```python
from build123d import *

# Parameters (mm, degrees)
BOSS_EXTRUDE1_DEPTH       = 12.7
FILLET1_R                 = 6.35
F_1_4_CLEARANCE_HOLE1_D   = 6.7564
TAP_DRILL_FOR_8_32_TAP1_D = 3.4544


with BuildPart() as part:
    # Sketch1 → Boss-Extrude1 (new body)
    with BuildSketch(Plane.XY):
        Polygon((12.7, 15.875), (31.75, 15.875), (31.75, 28.575), (-31.75, 28.575), (-31.75, 15.875), (-12.7, 15.875), (-12.7, -15.875), (12.7, -15.875), align=None)
    extrude(amount=BOSS_EXTRUDE1_DEPTH)

    # Fillet1
    fillet1_edges = [part.edges().sort_by_distance(p)[0] for p in [
        (-12.7, 15.875, 6.35),
        (12.7, 15.875, 6.35),
    ]]
    fillet(fillet1_edges, radius=FILLET1_R)

    # 1/4 Clearance Hole1 (through all)
    with Locations(Plane.XY.offset(12.7)):
        with Locations((0, -6.35), (0, 12.7)):
            Hole(F_1_4_CLEARANCE_HOLE1_D / 2)

    # Tap Drill for #8-32 Tap1 (through all)
    with Locations(Plane(origin=(0, 15.875, 0), x_dir=(-1, 0, 0), z_dir=(0, -1, 0))):
        with Locations((-25.4, -6.35), (25.4, -6.35)):
            Hole(TAP_DRILL_FOR_8_32_TAP1_D / 2)


solid = part.part
```
Read the model definition and answer for the solid it produces. Units are mm, in the model's axes. A direction names the side the tool comes from. Coordinates: 2 decimals unless noted, no trailing zeros. Loops run counter-clockwise (first coordinate to the right, second up) from the corner with the lowest first, then second, coordinate; pieces in that order, holes last.
(1) The part is cut by section B-B (z = 10.5). Determine the outline of the cut face in (x, y) (3 decimals), and give its area (3 significant figures).
Solution:
outline: (-31.75, 15.875) - (-19.05, 15.875) arc R6.35 cw to (-12.7, 9.525) - (-12.7, -15.875) - (12.7, -15.875) - (12.7, 9.525) arc R6.35 cw to (19.05, 15.875) - (31.75, 15.875) - (31.75, 28.575) - (-31.75, 28.575) - close; hole circle Ø6.756 at (0, -6.35); hole circle Ø6.756 at (0, 12.7)
area: 1,560 mm2
(2) The mould has two halves that part along X. Classify faces 4 (the face through (-14.61, 14.064, 6.439)), 5 (the face through (0, 17, 12.7)), 6 (the face through (26.329, 22.314, 4.894)): released by +X, released by -X, zero draft, split by the parting line, or undercut.
Solution:
face 4: released by -X
face 5: zero draft
face 6: undercut
(3) Flat-ended cylindrical pins translate along their axes: pin 1 Ø6.5 at (y, z) = (-1.5, 3.5) entering from -X; pin 2 Ø5.5 at (x, y) = (0, 12.7) entering from -Z; pin 3 Ø1 at (x, z) = (-23.5, 9) entering from -Y (3 decimals); pin 4 Ø11 at (x, y) = (0, -6.35) entering from +Z. Find the tip coordinate at first contact, or state that the pin passes through.
Solution:
pin 1: stops at x = -12.7
pin 2: passes through
pin 3: stops at y = 15.875
pin 4: stops at z = 12.7
(4) A tool of negligible diameter and unlimited length cuts with its end or side. For faces 1 (the face through (-27, 15.875, 8)), 2 (the face through (0.73, 9.4, 6.26)), 3 (the face through (24, 15.875, 8)), from which of +Z, -Z, +X, -X, +Y, -Y can it reach the whole face along a straight path? Write none if from no direction.
Solution:
face 1: +Z, -Z, -X, -Y
face 2: +Z, -Z
face 3: +Z, -Z, +X, -Y
(5) The part is cut by section D-D (y = 21). Determine the outline of the cut face in (x, z).
Solution:
outline: (-31.75, 0) - (31.75, 0) - (31.75, 12.7) - (-31.75, 12.7) - close; hole circle Ø3.45 at (-25.4, 6.35); hole circle Ø3.45 at (25.4, 6.35)
(6) Consider line 1 along Y through (x, z) = (0, 7.25) (3 decimals); line 2 along X through (y, z) = (24.25, 6.35); line 3 along Y through (x, z) = (1, 4) (3 decimals). Determine where each line is inside the solid, lowest interval first.
Solution:
line 1: y = -15.875 to -9.728, -2.972 to 9.322, 16.078 to 28.575
line 2: x = -31.75 to -27.13, -23.67 to 23.67, 27.13 to 31.75
line 3: y = -15.875 to -9.577, -3.123 to 9.473, 15.927 to 28.575
(7) The part is cut by section A-A (y = -6.35). Determine the outline of the cut face in (x, z).
Solution:
outline: (-12.7, 0) - (-3.38, 0) - (-3.38, 12.7) - (-12.7, 12.7) - close; (3.38, 0) - (12.7, 0) - (12.7, 12.7) - (3.38, 12.7) - close
(8) The part is cut by section C-C (x = 25.4). Determine the outline of the cut face in (y, z) (3 decimals), and give its area (3 significant figures).
Solution:
outline: (15.875, 0) - (28.575, 0) - (28.575, 4.623) - (15.875, 4.623) - close; (15.875, 8.077) - (28.575, 8.077) - (28.575, 12.7) - (15.875, 12.7) - close
area: 117 mm2
